from build123d import *

# Parameters (mm, degrees)
SKETCH1_R           = 6.3373
BOSS_EXTRUDE1_DEPTH = 38.1
CHAMFER1_SIZE       = 1.524
CHAMFER2_SIZE       = 1.524


with BuildPart() as part:
    # Sketch1 → Boss-Extrude1 (new body, symmetric)
    with BuildSketch(Plane(origin=(0, 0, 0), x_dir=(0, 0, -1), z_dir=(1, 0, 0))):
        Circle(SKETCH1_R)
    extrude(amount=BOSS_EXTRUDE1_DEPTH, both=True)

    # Chamfer1
    chamfer1_edges = [part.edges().sort_by_distance(p)[0] for p in [
        (38.1, 0, 6.3373),
    ]]
    chamfer(chamfer1_edges, length=CHAMFER1_SIZE)

    # Chamfer2
    chamfer2_edges = [part.edges().sort_by_distance(p)[0] for p in [
        (-38.1, 0, 6.3373),
    ]]
    chamfer(chamfer2_edges, length=CHAMFER2_SIZE)


solid = part.part
The model under review builds one solid part; all positions refer to its coordinate system, in mm. Give positions to 0.01 mm unless a question says otherwise; leave off trailing zeros. Write each loop counter-clockwise with the first axis right and the second up, starting at its lowest first coordinate (ties: lowest second). Pieces come first, ordered by that corner, then holes.
1. For P1, Ø1, axis at x = -10, z = 4.5, coming from the +Y side; P2, Ø4, axis at x = -18, y = -5, coming from the +Z side; P3, Ø6, axis at x = -24, z = 4.5, coming from the +Y side, all flat-tipped, find the tip position at first contact; note any pin that passes through.
2. Wall thickness on L1, parallel to Z at x = -28.5, y = 0.25; L2, parallel to X at y = 5.5, z = -2.75; L3, parallel to Y at x = -8.5, z = 3.25: over which ranges is each line inside the solid? List them lowest first.
3. Add section A-A, the plane x = -27. Write out the cut boundary in (y, z).
Worked answers:
1. P1: stops at y = 4.92
1. P2: stops at z = 5.58
1. P3: stops at y = 6.16
2. L1: z = -6.33 to 6.33
2. L2: x = -36.76 to 36.76
2. L3: y = -5.44 to 5.44
3. outline: circle Ø12.67 at (0, 0)
